```python
from build123d import *

# Parameters (mm, degrees)
SKETCH241_W     = 80
SKETCH241_H     = 70
PAD125_DEPTH    = 3
SKETCH242_R     = 1.6
POCKET081_DEPTH = 5
CHAMFER085_SIZE = 3
CHAMFER086_SIZE = 1


with BuildPart() as part:
    # Sketch241 → Pad125 (new body)
    with BuildSketch(Plane.XY):
        Rectangle(SKETCH241_W, SKETCH241_H)
    extrude(amount=PAD125_DEPTH)

    # Sketch242 → Pocket081 (cut)
    with BuildSketch(Plane.XY):
        with Locations((24, 27.5)):
            Circle(SKETCH242_R)
        with Locations((6, 27.5)):
            Circle(SKETCH242_R)
        with Locations((6, -27.5)):
            Circle(SKETCH242_R)
        with Locations((24, -27.5)):
            Circle(SKETCH242_R)
        with BuildLine():
            ThreePointArc((34.316718, 3.941209), (31, 0), (34.316718, -3.941209))
            Line((34.316718, -3.941209), (40, -4.926511))
            ThreePointArc((40, -4.926511), (45.854102, 0), (40, 4.926511))
            Line((40, 4.926511), (34.316718, 3.941209))
        make_face()
    pocket081 = extrude(amount=POCKET081_DEPTH, mode=Mode.SUBTRACT)

    # Mirrored016: Pocket081 across YZ
    add(pocket081.mirror(Plane.YZ), mode=Mode.SUBTRACT)

    # Chamfer085
    chamfer085_edges = [part.edges().sort_by_distance(p)[0] for p in [
        (-40, -35, 1.5),
        (40, -35, 1.5),
        (-40, 35, 1.5),
        (40, 35, 1.5),
    ]]
    chamfer(chamfer085_edges, length=CHAMFER085_SIZE)

    # Chamfer086
    chamfer086_edges = [part.edges().sort_by_distance(p)[0] for p in [
        (40, -4.926511, 1.5),
        (40, 4.926511, 1.5),
        (-40, 4.926511, 1.5),
        (-40, -4.926511, 1.5),
    ]]
    chamfer(chamfer086_edges, length=CHAMFER086_SIZE)


solid = part.part
```
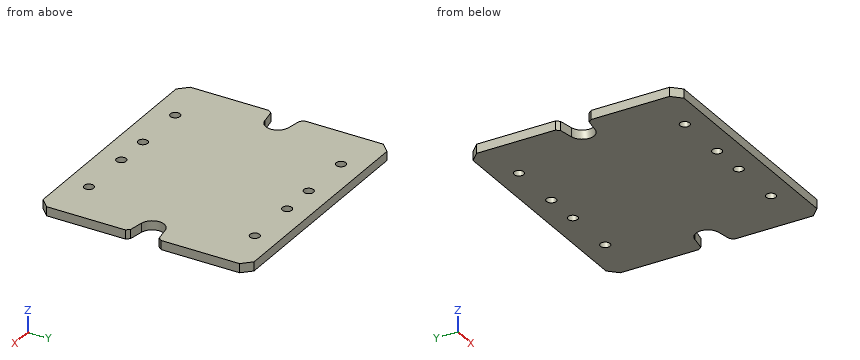
Input: part model. Units: mm. Frame: model coordinates. Coordinates: 2 decimals unless noted, no trailing zeros. Loops run counter-clockwise (first coordinate to the right, second up) from the corner with the lowest first, then second, coordinate; pieces in that order, holes last. Notation, with made-up numbers: M 55.5,-39.75 L 114.5,-39.75 A12 ccw 114.5,-35.75 Z; hole C 31.5,88.5 d4. An arc over 180 degrees is marked long. Use a Markdown table: item, result. Add a question column.
1) Pin query (flat end, axial travel): P1, Ø2.5, axis at x = -6, y = 27.5, coming from the +Z side. Return the tip coordinate at first contact, or that it passes through.
2) Line query: L1, parallel to Y at x = -6, z = 2.1; L2, parallel to X at y = 1, z = 1.9; L3, parallel to X at y = 2, z = 1.95. Output: solid intervals per line, ascending. Write a range as from..to.
3) Section C-C, the plane z = 2.15. Give the number of separate pieces and of enclosed holes in the cut face, plus the area to 3 significant figures.
4) Section B-B, the plane y = 27.5. Return the cut outline in (x, z).
5) Section A-A, the plane x = -24. Return the cut outline in (y, z), plus the area to 3 significant figures.
6) Section D-D, the plane x = 23.5. Return the cut outline in (y, z), plus the area to 3 significant figures.
Answer below:
| question | item | result |
|---|---|---|
| 1 | P1 | through |
| 2 | L1 | -35..-29.1, -25.9..25.9, 29.1..35 |
| 2 | L2 | -31.13..31.13 |
| 2 | L3 | -31.54..31.54 |
| 3 | separate pieces | 1 |
| 3 | enclosed holes | 8 |
| 3 | area | 5,380 mm2 |
| 4 | outline | M -40,0 L -25.6,0 L -25.6,3 L -40,3 Z; M -22.4,0 L -7.6,0 L -7.6,3 L -22.4,3 Z; M -4.4,0 L 4.4,0 L 4.4,3 L -4.4,3 Z; M 7.6,0 L 22.4,0 L 22.4,3 L 7.6,3 Z; M 25.6,0 L 40,0 L 40,3 L 25.6,3 Z |
| 5 | outline | M -35,0 L -29.1,0 L -29.1,3 L -35,3 Z; M -25.9,0 L 25.9,0 L 25.9,3 L -25.9,3 Z; M 29.1,0 L 35,0 L 35,3 L 29.1,3 Z |
| 5 | area | 191 mm2 |
| 6 | outline | M -35,0 L -29.02,0 L -29.02,3 L -35,3 Z; M -25.98,0 L 25.98,0 L 25.98,3 L -25.98,3 Z; M 29.02,0 L 35,0 L 35,3 L 29.02,3 Z |
| 6 | area | 192 mm2 |
